Geometry check sheet. Reference: drawing and pictorial views, mm from the part's lowest x, y, z. A direction names the side the tool comes from. Give positions to 0.01 mm unless a question says otherwise; leave off trailing zeros. Order: outer loops, then holes, each group sorted by start corner. A loop starts at its lowest first (then second) coordinate and runs counter-clockwise, first axis right, second up.
Item 1: Sectioned sample at D-D on x = 237. Record the boundary of the cut face in (y, z).
Item 2: Sectioned sample at B-B on y = 42. Record the boundary of the cut face in (x, z), and give its area (3 significant figures).
Item 3: Access from +Z, -Z, +X, -X, +Y, -Y to the whole of each face (thin tool, end or side, straight path). Record for the marked faces 1 and 2.
Item 4: Gauge pin test, flat end, axial feed: P1, Ø12, axis at x = 179.5, z = 214, coming from the +Y side. Record the tip position at first contact, or that the pin passes through.
Item 5: Release check for a two-part mould opening along Z. For the marked faces 3, 4 and 5 record: released by +Z, released by -Z, zero draft, split by the parting line, or undercut.
Item 6: Sectioned sample at A-A on x = 200. Record the boundary of the cut face in (y, z), and give its area (3 significant figures).
Item 7: Material ranges on line 1 along X through (y, z) = (36, 79); line 2 along Z through (x, y) = (110, 37); line 3 along X through (y, z) = (14.5, 122), recorded low to high.
Item 8: Sectioned sample at C-C on z = 122. Record the boundary of the cut face in (x, y).
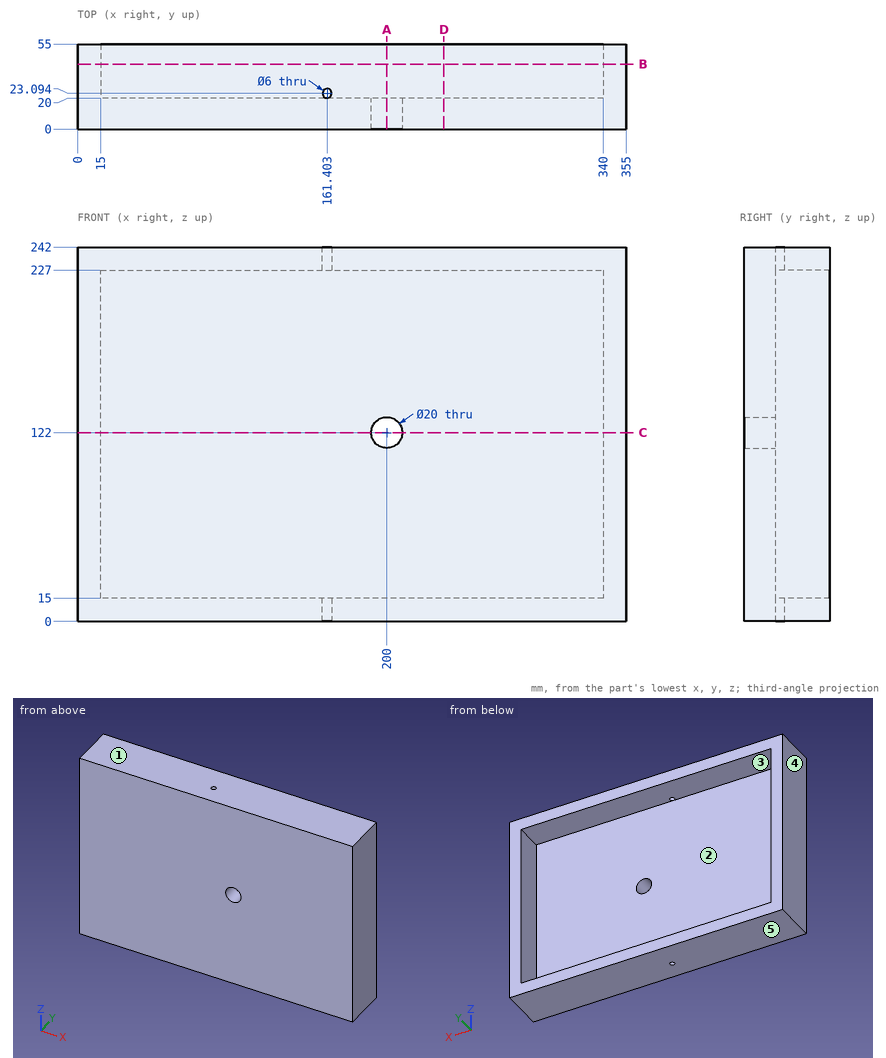
Report:
1. outline: (0, 0) - (55, 0) - (55, 15) - (20, 15) - (20, 227) - (55, 227) - (55, 242) - (0, 242) - close
2. outline: (0, 0) - (355, 0) - (355, 242) - (0, 242) - close; hole (15, 15) - (340, 15) - (340, 227) - (15, 227) - close
2. area: 17,000 mm2
3. face 1: +Z, +X, -X, +Y, -Y
3. face 2: +Y
4. P1: stops at y = 20
5. face 3: undercut
5. face 4: zero draft
5. face 5: released by -Z
6. outline: (0, 0) - (55, 0) - (55, 15) - (20, 15) - (20, 112) - (0, 112) - close; (0, 132) - (20, 132) - (20, 227) - (55, 227) - (55, 242) - (0, 242) - close
6. area: 5,490 mm2
7. line 1: x = 0 to 15, 340 to 355
7. line 2: z = 0 to 15, 227 to 242
7. line 3: x = 0 to 190, 210 to 355
8. outline: (0, 0) - (190, 0) - (190, 20) - (15, 20) - (15, 55) - (0, 55) - close; (210, 0) - (355, 0) - (355, 55) - (340, 55) - (340, 20) - (210, 20) - close
